Part model, mm, in its own coordinate system. A direction names the side the tool comes from. Round coordinates to 2 decimals unless told otherwise and drop trailing zeros. Loops run counter-clockwise (first coordinate to the right, second up) from the corner with the lowest first, then second, coordinate; pieces in that order, holes last.
from build123d import *

# Parameters (mm, degrees)
EXTRUDE_754_DEPTH              = 5
SKETCH_2_W                     = 10
SKETCH_2_H                     = 30
EXTRUDE_813_DEPTH              = 5
CHAMFER_861_SIZE               = 1.5
CHAMFER_861_OF_MIRROR_928_SIZE = 1.5
CUT_EXTRUDE_956_DEPTH          = 150.248115566
CUT_EXTRUDE_956_DEPTH_BACK     = 150.248115566
SKETCH_3_W                     = 74
SKETCH_3_H                     = 10.5
FILLET_R_R                     = 1


with BuildPart() as part:
    # ｽｹｯﾁ1 → Extrude 754 (new, symmetric)
    with BuildSketch(Plane(origin=(0, 0, 0), x_dir=(0, 0, -1), z_dir=(1, 0, 0))):
        with BuildLine():
            Line((75.5, 0), (105, 0))
            Line((105, 0), (105, -95))
            Line((105, -95), (-105, -95))
            Line((-105, -95), (-105, 0))
            Line((-105, 0), (-75.5, 0))
            ThreePointArc((-75.5, 0), (0, -75.5), (75.5, 0))
        make_face()
    extrude(amount=EXTRUDE_754_DEPTH, both=True)

    # ｽｹｯﾁ2 → Extrude 813 (add, symmetric)
    with BuildSketch(Plane(origin=(0, 0, 0), x_dir=(0, 0, -1), z_dir=(1, 0, 0))):
        with Locations((-110, -45)):
            Rectangle(SKETCH_2_W, SKETCH_2_H)
    extrude_813 = extrude(amount=EXTRUDE_813_DEPTH, both=True)

    # Chamfer 861
    chamfer_861_edges = [part.edges().sort_by_distance(p)[0] for p in [
        (0, -30, 115),
        (0, -60, 115),
    ]]
    chamfer(chamfer_861_edges, length=CHAMFER_861_SIZE)

    # Mirror 928: Extrude 813 across plane
    add(extrude_813.mirror(Plane.XY))

    # Chamfer 861 of Mirror 928
    chamfer_861_of_mirror_928_edges = [part.edges().sort_by_distance(p)[0] for p in [
        (0, -30, -115),
        (0, -60, -115),
    ]]
    chamfer(chamfer_861_of_mirror_928_edges, length=CHAMFER_861_OF_MIRROR_928_SIZE)

    # ｽｹｯﾁ3 → Cut-Extrude 956 (cut, two sides: drawn at the far end of the back side and taken through both)
    with BuildSketch(Plane(origin=(0, 0, 0), x_dir=(0, 0, -1), z_dir=(1, 0, 0)).offset(-CUT_EXTRUDE_956_DEPTH_BACK)):
        with Locations((0, -89.75)):
            Rectangle(SKETCH_3_W, SKETCH_3_H)
    extrude(amount=CUT_EXTRUDE_956_DEPTH + CUT_EXTRUDE_956_DEPTH_BACK, mode=Mode.SUBTRACT)

    # くぐり穴 内角R
    fillet_r_edges = [part.edges().sort_by_distance(p)[0] for p in [
        (0, -84.5, -37),
        (0, -84.5, 37),
    ]]
    fillet(fillet_r_edges, radius=FILLET_R_R)


solid = part.part
1) Drop flat-ended pins along their axis: pin 1 Ø4 at (x, z) = (-1.5, 10.5) entering from +Y; pin 2 Ø2.5 at (x, z) = (-2, 109) entering from +Y; pin 3 Ø4 at (x, z) = (-3, 19.5) entering from +Y. Give the stop position or say it passes through.
Values:
pin 1: stops at y = -74.46
pin 2: stops at y = -30
pin 3: stops at y = -72.37
2) Slice it at D-D, the plane y = -49. Give the cut face in (x, z).
Values:
outline: (-5, -115) - (5, -115) - (5, -57.44) - (-5, -57.44) - close; (-5, 57.44) - (5, 57.44) - (5, 115) - (-5, 115) - close
3) Tool access for faces 1 (the face through (0, -15, 105)), 2 (the face through (0, -60, -109)), 3 (the face through (0, -84.5, 1)): list every direction of +Z, -Z, +X, -X, +Y, -Y with a clear straight run to the whole face (end or side of a thin tool).
Values:
face 1: +Z, +X, -X, +Y
face 2: -Z, +X, -X, -Y
face 3: +X, -X, -Y
4) Slice it at B-B, the plane x = -1.25. Give the cut face in (y, z), then the cut area to 3 significant figures.
Values:
outline: (-95, -105) - (-60, -105) - (-60, -113.5) - (-58.5, -115) - (-31.5, -115) - (-30, -113.5) - (-30, -105) - (0, -105) - (0, -75.5) arc R75.5 cw to (0, 75.5) - (0, 105) - (-30, 105) - (-30, 113.5) - (-31.5, 115) - (-58.5, 115) - (-60, 113.5) - (-60, 105) - (-95, 105) - (-95, 37) - (-85.5, 37) arc R1 cw to (-84.5, 36) - (-84.5, -36) arc R1 cw to (-85.5, -37) - (-95, -37) - close
area: 10,800 mm2
5) Slice it at C-C, the plane z = 0. Give the cut face in (x, y), then the cut area to 3 significant figures.
Values:
outline: (-5, -84.5) - (5, -84.5) - (5, -75.5) - (-5, -75.5) - close
area: 90.0 mm2
6) Wall check: line 1 along Z through (x, y) = (3.5, -88.5); line 2 along Z through (x, y) = (1, -80); line 3 along Z through (x, y) = (-2, -65). Give the ranges that are in metal, low to high.
Values:
line 1: z = -105 to -37, 37 to 105
line 2: z = -105 to 105
line 3: z = -105 to -38.41, 38.41 to 105
7) Slice it at A-A, the plane y = -67. Give the cut face in (x, z), then the cut area to 3 significant figures.
Values:
outline: (-5, -105) - (5, -105) - (5, -34.8) - (-5, -34.8) - close; (-5, 34.8) - (5, 34.8) - (5, 105) - (-5, 105) - close
area: 1,400 mm2
